Model file for the job. Use its own axes, mm. Give positions to 0.01 mm unless a question says otherwise; leave off trailing zeros. Write each loop counter-clockwise with the first axis right and the second up, starting at its lowest first coordinate (ties: lowest second). Pieces come first, ordered by that corner, then holes.
```python
from build123d import *

# Parameters (mm, degrees)
F0_W    = 8.5
F0_H    = 79
F4_SIZE = 0.5


with BuildPart() as f1:
    # F0 (on Front) → F1 (revolve)
    with BuildSketch(Plane.XZ):
        with Locations((-4.25, 39.5)):
            Rectangle(F0_W, F0_H)
    revolve(axis=Axis((0, 0, 39.5), (0, 0, -1)))

    # F2 (on Front) → F3 (revolve, cut)
    with BuildSketch(Plane.XZ):
        Polygon((4.5, 67.5), (8.5, 67.5), (8.5, 71.5), align=None)
    revolve(axis=Axis((-1.373549, 0, 67.5), (1, 0, 0)), mode=Mode.SUBTRACT)

    # F4
    f4_edges = [f1.edges().sort_by_distance(p)[0] for p in [
        (8.5, 0, 79),
        (8.5, 0, 0),
    ]]
    chamfer(f4_edges, length=F4_SIZE)


solid = f1.part
```
1. Probe probe 1 along X at (y, z) = (0.5, 28); probe 2 along X at (y, z) = (-6.25, 4.5); probe 3 along Z at (x, y) = (4, -7). List the from-to ranges inside material, lowest first.
Calculated:
probe 1: x = -8.49 to 8.49
probe 2: x = -5.76 to 5.76
probe 3: z = 0.06 to 78.94
2. Pin check, flat tips, straight feed: P1, Ø2, axis at x = 6, z = 41, coming from the +Y side; P2, Ø6, axis at y = 3.5, z = 12.5, coming from the -X side; P3, Ø2, axis at x = 4.5, z = 14, coming from the -Y side. Stop position of each tip, or through.
Calculated:
P1: stops at y = 6.87
P2: stops at x = -8.49
P3: stops at y = -7.75
3. Pull direction Z, two halves, no side cores. Call faces 1 (the flat face through (0, 0, 79)), 2 (the flat face through (0, 0, 0)), 3 (the conical face through (6, 0, 69)): +Z half, -Z half, draft (parallel to the pull), parting line (faces both ways), or undercut.
Calculated:
face 1: +Z half
face 2: -Z half
face 3: undercut
4. Slice it at A-A, the plane z = 24. Write the cut outline in (x, y), and give its area (3 significant figures).
Calculated:
outline: circle Ø17 at (0, 0)
area: 227 mm2
